Work out the finished part from the listing and answer in its coordinate system (mm). Face numbers are marked on the shaded views. Round coordinates to 2 decimals unless told otherwise and drop trailing zeros. Write each loop counter-clockwise with the first axis right and the second up, starting at its lowest first coordinate (ties: lowest second). Pieces come first, ordered by that corner, then holes. Notation, with made-up numbers: M 74,45 L 94,45 A15 cw 94,61 Z; hole C 53.25,-23 d3. An arc over 180 degrees is marked long. One line per item, written item: value. Start each with the question number.
Q1. Given pin 1 Ø1 at (x, y) = (30, 22.5) entering from +Z; pin 2 Ø3 at (y, z) = (22, 19.5) entering from +X; pin 3 Ø1 at (x, y) = (16.5, 22.5) entering from -Z, each flat-ended and moving along its own axis, determine where each tip first touches the part or whether it passes through.
Q2. Find section C-C (y = 24.4). Write down the section's boundary in (x, z), and give its area (3 significant figures).
Q3. Find section B-B (z = 0). Write down the section's boundary in (x, y), and give its area (3 significant figures).
Q4. The mould has two halves that part along Z. Classify the marked faces 1 and 2: released by +Z, released by -Z, zero draft, split by the parting line, or undercut.
Q5. Consider probe 1 along Z at (x, y) = (0, 21); probe 2 along Z at (x, y) = (20, 22.25); probe 3 along X at (y, z) = (24.75, 35.5). Determine where each line is inside the solid, lowest interval first.
Q6. Find section A-A (x = 0). Write down the section's boundary in (y, z).
Q7. Find section D-D (x = -11). Write down the section's boundary in (y, z), and give its area (3 significant figures).
from build123d import *

# Parameters (mm, degrees)
SKETCH1_R                                        = 45.466
BOSS_EXTRUDE1_DEPTH                              = 25.4
SKETCH3_R                                        = 20.32
CUT_EXTRUDE1_DEPTH                               = 12.7
CSK_FOR_1_4_FLAT_HEAD_MACHINE_SCREW1_D           = 6.5278
CSK_FOR_1_4_FLAT_HEAD_MACHINE_SCREW1_DEPTH       = 25.4
CSK_FOR_1_4_FLAT_HEAD_MACHINE_SCREW1_CSINK_D     = 12.8778
CSK_FOR_1_4_FLAT_HEAD_MACHINE_SCREW1_CSINK_ANGLE = 82
CSK_FOR_1_4_FLAT_HEAD_MACHINE_SCREW1_TIP         = 1.961148974
SKETCH9_R                                        = 53.031918303
CUT_EXTRUDE3_DEPTH                               = 20.322357613


with BuildPart() as part:
    # Sketch1 → Boss-Extrude1 (new body)
    with BuildSketch(Plane(origin=(0, 0, 0), x_dir=(1, 0, 0), z_dir=(0, 1, 0))):
        Circle(SKETCH1_R)
    extrude(amount=BOSS_EXTRUDE1_DEPTH)

    # Sketch3 → Cut-Extrude1 (cut)
    with BuildSketch(Plane.XZ):
        Circle(SKETCH3_R)
    extrude(amount=-CUT_EXTRUDE1_DEPTH, mode=Mode.SUBTRACT)

    # CSK for 1/4 Flat Head Machine Screw1
    with Locations(Plane(origin=(0, 25.4, 0), x_dir=(1, 0, 0), z_dir=(0, 1, 0))):
        with Locations((0, 0)):
            CounterSinkHole(CSK_FOR_1_4_FLAT_HEAD_MACHINE_SCREW1_D / 2, CSK_FOR_1_4_FLAT_HEAD_MACHINE_SCREW1_CSINK_D / 2, depth=CSK_FOR_1_4_FLAT_HEAD_MACHINE_SCREW1_DEPTH, counter_sink_angle=CSK_FOR_1_4_FLAT_HEAD_MACHINE_SCREW1_CSINK_ANGLE)
            with Locations((0, 0, -(CSK_FOR_1_4_FLAT_HEAD_MACHINE_SCREW1_DEPTH + CSK_FOR_1_4_FLAT_HEAD_MACHINE_SCREW1_TIP / 2))):  # 118° drill point
                Cone(0, CSK_FOR_1_4_FLAT_HEAD_MACHINE_SCREW1_D / 2, CSK_FOR_1_4_FLAT_HEAD_MACHINE_SCREW1_TIP, mode=Mode.SUBTRACT)

    # Sketch9 → Cut-Extrude3 (cut)
    with BuildSketch(Plane.XZ):
        Circle(SKETCH9_R)
    extrude(amount=-CUT_EXTRUDE3_DEPTH, mode=Mode.SUBTRACT)


solid = part.part
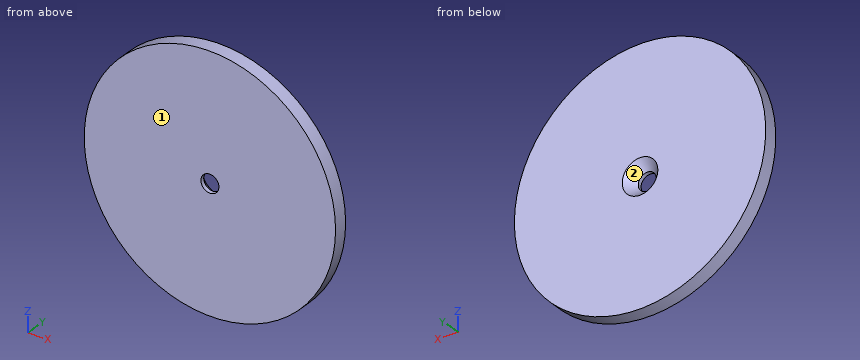
The answers:
1. pin 1: z = 34.6
1. pin 2: x = 41.75
1. pin 3: z = -42.56
2. outline: C 0,0 d90.93; hole C 0,0 d11.14
2. area: 6,400 mm2
3. outline: M -45.47,20.32 L -3.26,20.32 L -3.26,21.75 L -6.44,25.4 L -45.47,25.4 Z; M 3.26,20.32 L 45.47,20.32 L 45.47,25.4 L 6.44,25.4 L 3.26,21.75 Z
3. area: 417 mm2
4. face 1: zero draft
4. face 2: undercut
5. probe 1: -45.47 to -3.26, 3.26 to 45.47
5. probe 2: -40.83 to 40.83
5. probe 3: -28.41 to 28.41
6. outline: M 20.32,-45.47 L 25.4,-45.47 L 25.4,-6.44 L 21.75,-3.26 L 20.32,-3.26 Z; M 20.32,3.26 L 21.75,3.26 L 25.4,6.44 L 25.4,45.47 L 20.32,45.47 Z
7. outline: M 20.32,-44.12 L 25.4,-44.12 L 25.4,44.12 L 20.32,44.12 Z
7. area: 448 mm2
